Autodesk Inventor part; units mm, degrees
ref_plane "YZ Plane" through (0, 0, 0) normal (1, 0, 0) x (0, 1, 0)
ref_plane "XZ Plane" through (0, 0, 0) normal (0, 1, 0) x (-1, 0, 0)
ref_plane "XY Plane" through (0, 0, 0) normal (0, 0, 1) x (1, 0, 0)
sketch "スケッチ1" plane through (0, 0, 0) normal (0, 0, 1) x (1, 0, 0)
  circle A0 centre (0, 0) radius 30
  circle A1 centre (0, 0) radius 6
  dimension "d0" = 12
  dimension "d1" = 60
extrude "押し出し1" add sketch "スケッチ1" along normal mid plane 32
sketch "スケッチ3" plane through (0, 0, 16) normal (0, 0, 1) x (1, 0, 0)
  circle A0 centre (0, 0) radius 11.5 construction
  circle A1 centre (-9.9593, 5.75) radius 1.6
  circle A2 centre (0, -11.5) radius 1.6
  circle A3 centre (9.9593, 5.75) radius 1.6
  dimension "d7" = 23
  dimension "d8" = 3.2
  dimension "d11" = 360
extrude "押し出し3" cut sketch "スケッチ3" against normal through all
sketch "スケッチ2" plane through (0, 0, 16) normal (0, 0, 1) x (1, 0, 0)
  circle A0 centre (0, 0) radius 7
  dimension "d4" = 14
extrude "押し出し2" cut sketch "スケッチ2" against normal blind 2
mirror "ミラー1" about plane through (0, 0, 0) normal (0, 0, 1) of "押し出し2"
properties part number "mecanumL"
The model under review builds one solid part; all positions refer to its coordinate system, in mm. A direction names the side the tool comes from. Give positions to 0.01 mm unless a question says otherwise; leave off trailing zeros. Order: outer loops, then holes, each group sorted by start corner. A loop starts at its lowest first (then second) coordinate and runs counter-clockwise, first axis right, second up. Notation, with made-up numbers: M 72.25,-6.75 L 117.25,-6.75 A14 ccw 117.25,17.25 Z; hole C -1.75,-31.5 d1. An arc over 180 degrees is marked long. Answer in a Markdown table with one row per item. Add a question column.
1. Add section C-C on z = 5. State the section outline as (x, y) points.
2. Add section B-B on y = 0. State the section outline as (x, z) points.
3. To check wall thickness, follow line 1 along Y through (x, z) = (0, 1.5); line 2 along Y through (x, z) = (0, 14.9); line 3 along Y through (x, z) = (4, -5.5). State the ranges of each line that lie inside material, in increasing order.
4. Add section A-A on x = 0. State the section outline as (y, z) points.
5. Machinability: for faces 1 (the cylindrical face through (6.466, -2.681, 15.014)), 2 (the cylindrical face through (6.466, 2.681, -15.014)), 3 (the flat face through (6, -6, 16)), which of the approach directions +Z, -Z, +X, -X, +Y, -Y give a long, thin tool a straight path to every point of the face, cutting with its end or side? Answer none if there is none.
6. For pin 1 Ø5 at (x, y) = (-9.96, 5.75) entering from -Z; pin 2 Ø3 at (x, z) = (-1.5, 6) entering from +Y; pin 3 Ø10 at (y, z) = (21, -6) entering from -X; pin 4 Ø8.5 at (x, y) = (0, 0) entering from +Z, all flat-tipped, find the tip position at first contact; note any pin that passes through.
7. Add section D-D on y = -11.5. State the section outline as (x, z) points.
8. Mouldability with a two-part tool opening along X and no side actions: class faces 4 (the flat face through (-6, 2, -14)), 5 (the flat face through (6, -6, -16)), 6 (the cylindrical face through (-29.97, 1.32, 0.22)), 7 (the flat face through (6, 2, 14)) as released by +X, released by -X, zero draft, split by the parting line, or undercut.
The answers:
| question | item | result |
|---|---|---|
| 1 | outline | C 0,0 d60; hole C -9.96,5.75 d3.2; hole C 0,0 d12; hole C 0,-11.5 d3.2; hole C 9.96,5.75 d3.2 |
| 2 | outline | M -30,-16 L -7,-16 L -7,-14 L -6,-14 L -6,14 L -7,14 L -7,16 L -30,16 Z; M 6,-14 L 7,-14 L 7,-16 L 30,-16 L 30,16 L 7,16 L 7,14 L 6,14 Z |
| 3 | line 1 | -30 to -13.1, -9.9 to -6, 6 to 30 |
| 3 | line 2 | -30 to -13.1, -9.9 to -7, 7 to 30 |
| 3 | line 3 | -29.73 to -4.47, 4.47 to 29.73 |
| 4 | outline | M -30,-16 L -13.1,-16 L -13.1,16 L -30,16 Z; M -9.9,-16 L -7,-16 L -7,-14 L -6,-14 L -6,14 L -7,14 L -7,16 L -9.9,16 Z; M 6,-14 L 7,-14 L 7,-16 L 30,-16 L 30,16 L 7,16 L 7,14 L 6,14 Z |
| 5 | face 1 | +Z |
| 5 | face 2 | -Z |
| 5 | face 3 | +Z, +X, -X, +Y, -Y |
| 6 | pin 1 | z = -16 |
| 6 | pin 2 | y = 30 |
| 6 | pin 3 | x = -25.38 |
| 6 | pin 4 | through |
| 7 | outline | M -27.71,-16 L -1.6,-16 L -1.6,16 L -27.71,16 Z; M 1.6,-16 L 27.71,-16 L 27.71,16 L 1.6,16 Z |
| 8 | face 4 | undercut |
| 8 | face 5 | zero draft |
| 8 | face 6 | split by the parting line |
| 8 | face 7 | undercut |
